Source: CAD feature listing. Evaluate the final solid. Frame: model axes, mm. Face numbers are marked on the shaded views. Coordinates: 2 decimals unless noted, no trailing zeros. Write each loop counter-clockwise with the first axis right and the second up, starting at its lowest first coordinate (ties: lowest second). Pieces come first, ordered by that corner, then holes. Notation, with made-up numbers: (-27, -18) -> (13, -18) arc R21 cw to (13, -11) -> close; hole circle Ø7 at (-36.5, 76). An arc over 180 degrees is marked (long way). One line per item, written item: value. Start each with the question number.
1. Line query: line 1 (Y direction, x = 9.25, z = 0); line 2 (Z direction, x = 6.25, y = 4); line 3 (Z direction, x = 4.25, y = 1). Output: solid intervals per line, ascending.
2. Mould query, pull axis Z, two halves, no side actions, for the marked faces 1, 2 and 3. Classes: released by +Z, released by -Z, zero draft, split by the parting line, or undercut.
3. First-contact query: P1, Ø1, axis at x = 2, z = -9.5, coming from the +Y side; P2, Ø12, axis at x = 11, z = 6, coming from the +Y side; P3, Ø6, axis at x = 14, y = 6.5, coming from the +Z side; P4, Ø5, axis at x = 12, y = 3.5, coming from the +Z side. Flat tips, straight axial feed; report the tip coordinate or a pass-through.
4. Section query C-C, the plane y = 3. Output: boundary loops of the cut face in (x, z).
5. Section query A-A, the plane z = 0. Output: boundary loops of the cut face in (x, y).
6. Section query B-B, the plane x = 9. Output: boundary loops of the cut face in (y, z).
from build123d import *

# Parameters (mm, degrees)
CYLINDER_R              = 10.1
CYLINDER_DEPTH          = 20
CYLINDER_PITCH_ANGLE    = 90
CYLINDER001_R           = 12
CYLINDER001_DEPTH       = 22
CYLINDER001_PITCH_ANGLE = 90


with BuildPart() as cylinder:
    # Cylinder → Cylinder (new body)
    with BuildSketch(Plane.XY):
        Circle(CYLINDER_R)
    extrude(amount=CYLINDER_DEPTH)


with BuildPart() as cylinder_1:
    # Cylinder pitch: moved
    add(cylinder.part.rotate(Axis((0, 0, 0), (0, 1, 0)), CYLINDER_PITCH_ANGLE))


with BuildPart() as cylinder_2:
    # Cylinder placement: moved
    add(cylinder_1.part)


with BuildPart() as cut:
    # Cylinder001 → Cylinder001 (new body)
    with BuildSketch(Plane.XY):
        Circle(CYLINDER001_R)
    extrude(amount=CYLINDER001_DEPTH)


with BuildPart() as cut_1:
    # Cylinder001 pitch: moved
    add(cut.part.rotate(Axis((0, 0, 0), (0, 1, 0)), CYLINDER001_PITCH_ANGLE))


with BuildPart() as cut_2:
    # Cylinder001 placement: moved
    add(cut_1.part.moved(Location((-2, 0, 0))))

    # Cut: cut Cylinder
    add(cylinder_2.part, mode=Mode.SUBTRACT)


solid = cut_2.part
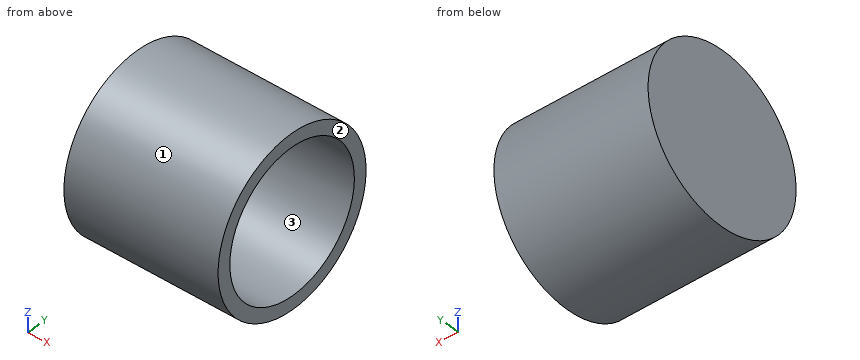
Computed values:
1. line 1: y = -12 to -10.1, 10.1 to 12
1. line 2: z = -11.31 to -9.27, 9.27 to 11.31
1. line 3: z = -11.96 to -10.05, 10.05 to 11.96
2. face 1: split by the parting line
2. face 2: zero draft
2. face 3: undercut
3. P1: stops at y = 7.94
3. P2: stops at y = 12
3. P3: stops at z = 11.48
3. P4: stops at z = 11.96
4. outline: (-2, -11.62) -> (20, -11.62) -> (20, -9.64) -> (0, -9.64) -> (0, 9.64) -> (20, 9.64) -> (20, 11.62) -> (-2, 11.62) -> close
5. outline: (-2, -12) -> (20, -12) -> (20, -10.1) -> (0, -10.1) -> (0, 10.1) -> (20, 10.1) -> (20, 12) -> (-2, 12) -> close
6. outline: circle Ø24 at (0, 0); hole circle Ø20.2 at (0, 0)
